Read the model definition and answer for the solid it produces. Units are mm, in the model's axes. A direction names the side the tool comes from. Give positions to 0.01 mm unless a question says otherwise; leave off trailing zeros. Write each loop counter-clockwise with the first axis right and the second up, starting at its lowest first coordinate (ties: lowest second). Pieces come first, ordered by that corner, then holes. Notation, with made-up numbers: (84, 15.25) -> (126, 15.25) arc R31 ccw to (126, 42.25) -> close; hole circle Ø5 at (24, 8). An arc over 180 degrees is marked (long way). Write item = value, one per line.
from build123d import *

# Parameters (mm, degrees)
SKETCH1_R           = 12.5
BOSS_EXTRUDE1_DEPTH = 10


with BuildPart() as part:
    # Sketch1 → Boss-Extrude1 (new body)
    with BuildSketch(Plane(origin=(0, 0, 0), x_dir=(1, 0, 0), z_dir=(0, 1, 0))):
        Circle(SKETCH1_R)
        Polygon((50, 100), (0, 0), (0, 100), align=None)
        Polygon((-111.602540378, -6.698729811), (0, 0), (-86.602540378, -50), align=None)
        Polygon((61.602540378, -93.301270189), (0, 0), (86.602540378, -50), align=None)
        with BuildLine():
            Line((-12.477543337, -0.748940761), (0, 0))
            Line((0, 0), (0, 12.5))
            ThreePointArc((0, 12.5), (-9.09977361, 8.569954507), (-12.477543337, -0.748940761))
        make_face()
        with BuildLine():
            Line((0, 12.5), (0, 0))
            Line((0, 0), (5.590169944, 11.180339887))
            ThreePointArc((5.590169944, 11.180339887), (2.871911507, 12.165612368), (0, 12.5))
        make_face()
        with BuildLine():
            Line((5.590169944, 11.180339887), (0, 0))
            Line((0, 0), (10.825317547, -6.25))
            ThreePointArc((10.825317547, -6.25), (12.074072829, -3.235238064), (12.5, 0))
            ThreePointArc((12.5, 0), (10.633135104, 6.571638901), (5.590169944, 11.180339887))
        make_face()
        with BuildLine():
            Line((10.825317547, -6.25), (0, 0))
            Line((0, 0), (6.887373394, -10.431399127))
            ThreePointArc((6.887373394, -10.431399127), (9.09977361, -8.569954507), (10.825317547, -6.25))
        make_face()
        with BuildLine():
            Line((6.887373394, -10.431399127), (0, 0))
            Line((0, 0), (-10.825317547, -6.25))
            ThreePointArc((-10.825317547, -6.25), (-2.871911507, -12.165612368), (6.887373394, -10.431399127))
        make_face()
        with BuildLine():
            Line((-10.825317547, -6.25), (0, 0))
            Line((0, 0), (-12.477543337, -0.748940761))
            ThreePointArc((-12.477543337, -0.748940761), (-11.971685117, -3.595657862), (-10.825317547, -6.25))
        make_face()
    extrude(amount=BOSS_EXTRUDE1_DEPTH)


solid = part.part
(1) The part is cut by section C-C on z = -59. Determine the outline of the cut face in (x, y), plus the area to 3 significant figures.
Checks:
outline = (0, 0) -> (29.5, 0) -> (29.5, 10) -> (0, 10) -> close
area = 295 mm²
(2) Consider L1, parallel to Z at x = 23.5, y = 2; L2, parallel to Z at x = 47, y = 5; L3, parallel to Z at x = -79, y = 5. Determine where each line is inside the solid, lowest interval first.
Checks:
L1 = -100 to -47, 13.57 to 35.59
L2 = -100 to -94, 27.14 to 71.18
L3 = 4.74 to 45.61
(3) A tool of negligible diameter and unlimited length cuts with its end or side. For faces 1 (the flat face through (28, 5, -56)), 2 (the flat face through (74.278, 4.93, 71.348)), 3 (the flat face through (0, 5, -56)), from which of +Z, -Z, +X, -X, +Y, -Y can it reach the whole face along a straight path? Write none if from no direction.
Checks:
face_1 = +X, +Y, -Y
face_2 = +Z, +X, +Y, -Y
face_3 = -Z, -X, +Y, -Y
(4) The part is cut by section D-D on x = 15.5. Determine the outline of the cut face in (y, z).
Checks:
outline = (0, -100) -> (10, -100) -> (10, -31) -> (0, -31) -> close; (0, 8.95) -> (10, 8.95) -> (10, 23.48) -> (0, 23.48) -> close
(5) For a pull along X with two mould halves and no side action, classify faces 4 (the flat face through (2, 10, -4)), 5 (the flat face through (-48.183, 4.93, 27.819)), 6 (the flat face through (34.63, 4.93, 52.45)), 7 (the flat face through (48.183, 4.93, 27.819)) as released by +X, released by -X, zero draft, split by the parting line, or undercut.
Checks:
face_4 = zero draft
face_5 = undercut
face_6 = undercut
face_7 = released by +X
(6) The part is cut by section B-B on y = 2.75. Determine the outline of the cut face in (x, z).
Checks:
outline = (-111.6, 6.7) -> (-12.48, 0.75) arc R12.5 ccw to (0, -12.5) -> (0, -100) -> (50, -100) -> (5.59, -11.18) arc R12.5 ccw to (10.83, 6.25) -> (86.6, 50) -> (61.6, 93.3) -> (6.89, 10.43) arc R12.5 ccw to (-10.83, 6.25) -> (-86.6, 50) -> close
(7) Given P1, Ø1.5, axis at y = 4, z = 2.5, coming from the +X side; P2, Ø5, axis at x = -22, y = 7, coming from the +Z side; P3, Ø5, axis at y = 5.5, z = -61.5, coming from the -X side, each flat-ended and moving along its own axis, determine where each tip first touches the part or whether it passes through.
Checks:
P1 = 12.38
P2 = 14.15
P3 = 0
(8) The part is cut by section A-A on x = 45. Determine the outline of the cut face in (y, z).
Checks:
outline = (0, -100) -> (10, -100) -> (10, -90) -> (0, -90) -> close; (0, 25.98) -> (10, 25.98) -> (10, 68.16) -> (0, 68.16) -> close
